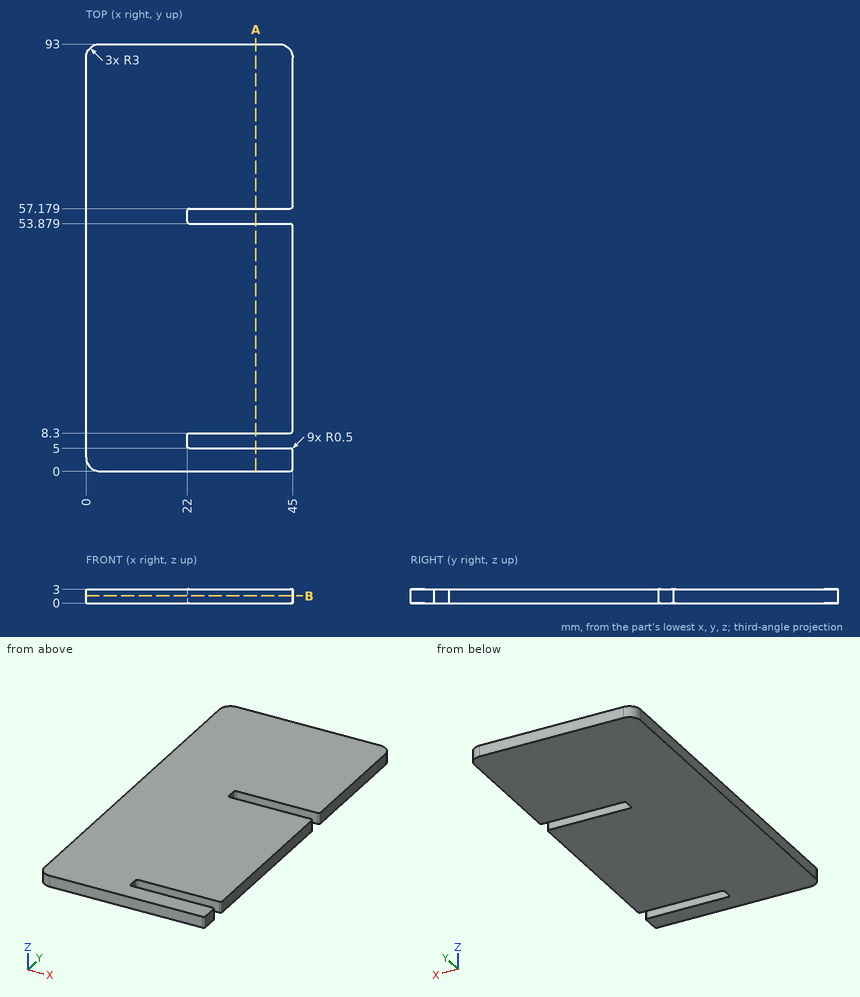
Answer from the drawing. Dimensions are ordinates in mm from the lowest x, y and z of the part. Coordinates: 2 decimals unless noted, no trailing zeros. Loops run counter-clockwise (first coordinate to the right, second up) from the corner with the lowest first, then second, coordinate; pieces in that order, holes last. Notation, with made-up numbers: (-14.75, 73.5) -> (4.25, 73.5) arc R11 ccw to (4.25, 94.5) -> close; hole circle Ø11 at (-37.75, 2). An arc over 180 degrees is marked (long way). Return JSON: item names as keys, results as strings.
Item 1: Find the intervals of material crossed by probe 1 along Y at (x, z) = (37.5, 1.2); probe 2 along X at (y, z) = (54, 0.65) (1 decimal), in increasing order.
Answers:
{"probe 1": "y = 0 to 5, 8.3 to 53.88, 57.18 to 93", "probe 2": "x = 0 to 22.2"}
Item 2: Find section A-A (x = 37). Determine the outline of the cut face in (y, z).
Answers:
{"outline": "(0, 0) -> (5, 0) -> (5, 3) -> (0, 3) -> close; (8.3, 0) -> (53.88, 0) -> (53.88, 3) -> (8.3, 3) -> close; (57.18, 0) -> (93, 0) -> (93, 3) -> (57.18, 3) -> close"}
Item 3: Find section B-B (z = 1.55). Determine the outline of the cut face in (x, y), plus the area to 3 significant figures.
Answers:
{"outline": "(0, 3) arc R3 ccw to (3, 0) -> (44.5, 0) arc R0.5 ccw to (45, 0.5) -> (45, 4.5) arc R0.5 ccw to (44.5, 5) -> (22.5, 5) arc R0.5 cw to (22, 5.5) -> (22, 7.8) arc R0.5 cw to (22.5, 8.3) -> (44.5, 8.3) arc R0.5 ccw to (45, 8.8) -> (45, 53.38) arc R0.5 ccw to (44.5, 53.88) -> (22.5, 53.88) arc R0.5 cw to (22, 54.38) -> (22, 56.68) arc R0.5 cw to (22.5, 57.18) -> (44.5, 57.18) arc R0.5 ccw to (45, 57.68) -> (45, 90) arc R3 ccw to (42, 93) -> (3, 93) arc R3 ccw to (0, 90) -> close", "area": "4,030 mm2"}
Item 4: A flat-ended cylindrical pin translates along its axis: P1, Ø0.7, axis at y = 55.5, z = 1, coming from the +X side. Find the tip coordinate at first contact, or state that the pin passes through.
Answers:
{"P1": "stops at x = 22"}
